Check sheet for the drawn part. Datum: minimum x, y, z corner. Units: mm. Coordinates: 2 decimals unless noted, no trailing zeros. Order: outer loops, then holes, each group sorted by start corner. A loop starts at its lowest first (then second) coordinate and runs counter-clockwise, first axis right, second up. Notation, with made-up numbers: (55.5, 62) - (84.5, 62) arc R27 cw to (84.5, 92) - close; hole circle Ø4 at (51.25, -16). An arc over 180 degrees is marked (long way). Put each result on its own line as item: value.
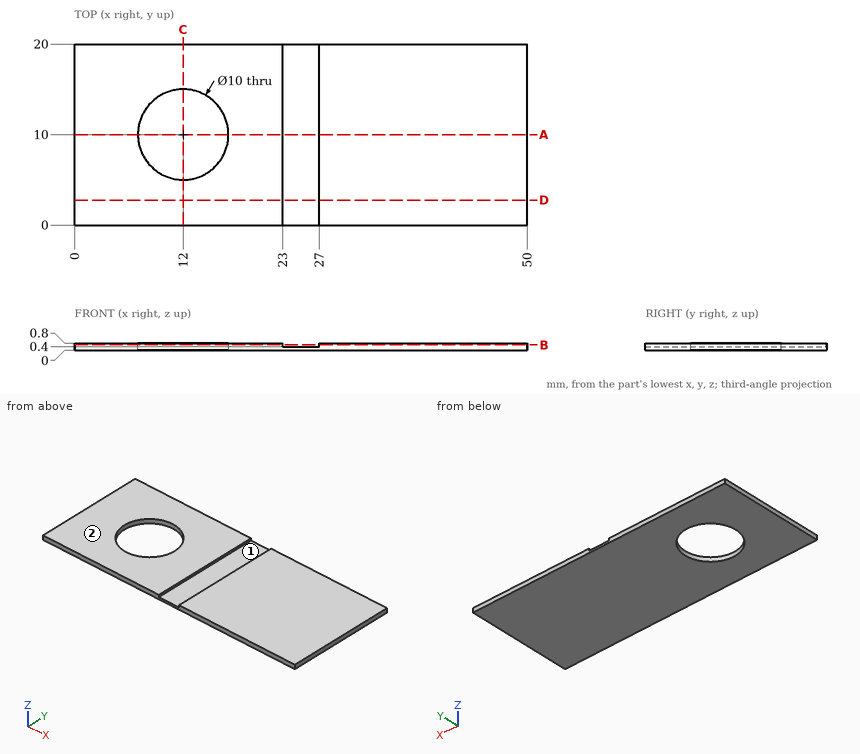
Q1. Draft check along X on the marked faces 1 and 2. Enter one of: pulls with the +X half, pulls with the -X half, needs draft (parallel to the pull), parting line crosses it, or undercut.
Answer block:
face 1: undercut
face 2: needs draft
Q2. Section check B-B on z = 0.6. Record the boundary of the cut face in (x, y).
Answer block:
outline: (0, 0) - (23, 0) - (23, 20) - (0, 20) - close; (27, 0) - (50, 0) - (50, 20) - (27, 20) - close; hole circle Ø10 at (12, 10)
Q3. Depth check by flat-ended pin: pin 1 Ø1.2 at (x, y) = (25.5, 11.5) entering from +Z. Enter the tip coordinate at first touch or a pass-through.
Answer block:
pin 1: stops at z = 0.4
Q4. Section check D-D on y = 2.75. Record the boundary of the cut face in (x, z), then the cut area to 3 significant figures.
Answer block:
outline: (0, 0) - (50, 0) - (50, 0.8) - (27, 0.8) - (27, 0.4) - (23, 0.4) - (23, 0.8) - (0, 0.8) - close
area: 38.4 mm^2
Q5. Section check A-A on y = 10. Record the boundary of the cut face in (x, z), then the cut area to 3 significant figures.
Answer block:
outline: (0, 0) - (7, 0) - (7, 0.8) - (0, 0.8) - close; (17, 0) - (50, 0) - (50, 0.8) - (27, 0.8) - (27, 0.4) - (23, 0.4) - (23, 0.8) - (17, 0.8) - close
area: 30.4 mm^2
Q6. Section check C-C on x = 12. Record the boundary of the cut face in (y, z), then the cut area to 3 significant figures.
Answer block:
outline: (0, 0) - (5, 0) - (5, 0.8) - (0, 0.8) - close; (15, 0) - (20, 0) - (20, 0.8) - (15, 0.8) - close
area: 8.00 mm^2
Q7. Thickness scan on L1, parallel to Y at x = 12, z = 0.45; L2, parallel to X at y = 7.5, z = 0.45; L3, parallel to X at y = 14.5, z = 0.6. Record the ranges inside material, lowest first. Write a range as [from, to].
Answer block:
L1: y = [0, 5], [15, 20]
L2: x = [0, 7.67], [16.33, 23], [27, 50]
L3: x = [0, 9.82], [14.18, 23], [27, 50]
